Here's how the part is built. I have some questions about the finished solid (model axes, mm). A direction names the side the tool comes from. Round coordinates to 2 decimals unless told otherwise and drop trailing zeros. Order: outer loops, then holes, each group sorted by start corner. A loop starts at its lowest first (then second) coordinate and runs counter-clockwise, first axis right, second up. Notation, with made-up numbers: (-3.5, -14.5) -> (20.5, -14.5) arc R14 ccw to (20.5, -2.5) -> close; hole circle Ø4 at (49, 14.25). An arc over 180 degrees is marked (long way). Use a Markdown table: item, result. Add a question column.
from build123d import *

# Parameters (mm, degrees)
F0_W     = 600
F0_H     = 600
F0_W_2   = 500
F0_H_2   = 500
F1_DEPTH = 30
F4_W     = 50
F4_H     = 50
F2_W     = 50
F2_H     = 50
F7_W     = 50
F7_H     = 50
F6_W     = 50
F6_H     = 50


with BuildPart() as f1:
    # F0 (on Top) → F1 (new body)
    with BuildSketch(Plane.XY):
        Rectangle(F0_W, F0_H)
        Rectangle(F0_W_2, F0_H_2, mode=Mode.SUBTRACT)
        Rectangle(F0_W_2, F0_H_2)
    extrude(amount=F1_DEPTH)

    # F4 (on offset) → F5 section 0
    with BuildSketch(Plane.XY.offset(800)):
        with Locations((-300, 300)):
            Rectangle(F4_W, F4_H)
    # F2 (on face) → F5 section 1
    with BuildSketch(Plane.XY.offset(30)):
        with Locations((-225, 225)):
            Rectangle(F2_W, F2_H)
    loft()

    # F7 (on offset) → F8 section 0
    with BuildSketch(Plane.XY.offset(800)):
        with Locations((300, 300)):
            Rectangle(F7_W, F7_H)
    # F6 (on face) → F8 section 1
    with BuildSketch(Plane.XY.offset(30)):
        with Locations((225, 225)):
            Rectangle(F6_W, F6_H)
    loft()

    # F9: F1 across plane


with BuildPart() as f1_1:
    add(f1.part)
    add(f1.part.mirror(Plane.XZ))


solid = f1_1.part
(1) I'm going to push flat-ended pins straight in: P1, Ø10, axis at x = -58, y = -235, coming from the +Z side; P2, Ø15, axis at x = 90, z = 11, coming from the +Y side; P3, Ø24, axis at y = 149, z = 10.5, coming from the -X side. Where does each tip first touch, or does it pass through?
(2) Please list where these lines run through material, in increasing order: probe 1 along Z at (x, y) = (-31, 81); probe 2 along X at (y, z) = (-267.5, 271); probe 3 along Y at (x, z) = (229, 227.5). Write a range as from..to.
(3) I want a section at A-A on x = -260. State how many separate pieces and enclosed holes the cut face has, and give its area (3 significant figures).
(4) I want a section at B-B on y = 176.5. List the corners of the cut face in (x, z) for me.
(5) On a 3-axis mill with a long thin cutter (end or side, diameter ignored), from which of +Z, -Z, +X, -X, +Y, -Y can I reach the whole of each face in a straight line? I mean faces 1 (the flat face through (-4, -300, 15)), 2 (the flat face through (300, -4, 15)), 3 (the flat face through (-4, 300, 15)), 4 (the flat face through (-300, -4, 15)). Say none if no direction works.
Output:
| question | item | result |
|---|---|---|
| 1 | P1 | z = 30 |
| 1 | P2 | y = 300 |
| 1 | P3 | x = -300 |
| 2 | probe 1 | 0..30 |
| 2 | probe 2 | -273.47..-223.47, 223.47..273.47 |
| 2 | probe 3 | -269.24..-219.24, 219.24..269.24 |
| 3 | separate pieces | 3 |
| 3 | enclosed holes | 0 |
| 3 | area | 69,300 mm² |
| 4 | outline | (-300, 0) -> (300, 0) -> (300, 30) -> (-300, 30) -> close |
| 5 | face 1 | -Z, +X, -X, -Y |
| 5 | face 2 | -Z, +X, +Y, -Y |
| 5 | face 3 | -Z, +X, -X, +Y |
| 5 | face 4 | -Z, -X, +Y, -Y |
